CAD build for the part. Positions are in the model's coordinates, mm. A direction names the side the tool comes from. Give positions to 0.01 mm unless a question says otherwise; leave off trailing zeros. Write each loop counter-clockwise with the first axis right and the second up, starting at its lowest first coordinate (ties: lowest second). Pieces come first, ordered by that corner, then holes. Notation, with made-up numbers: (62, -9) - (75, -9) arc R26 cw to (75, 7) - close; hole circle Ø2 at (58, 22.25). An arc over 180 degrees is marked (long way). Put each result on its own line as item: value. Start each with the question number.
1. Cut at B-B on x = 16.25. List the corners of the cut face in (y, z).
2. Wall check: line 1 (Z direction, x = 14, y = 4); line 2 (Z direction, x = 14, y = 2); line 3 (X direction, y = 4, z = 29.25). Give the ranges that are in metal, low to high.
3. Cut at D-D on y = 4. List the corners of the cut face in (x, z), and give its area (4 significant figures).
4. Cut at A-A on y = 0.25. List the corners of the cut face in (x, z), and give its area (4 significant figures).
5. Mould opens along Y. For faces 5 (the flat face through (17.25, 4, 22)), 6 (the flat face through (15, 2, 28)), 7 (the flat face through (16, 4, 33)) say: +Y half, -Y half, draft (parallel to the pull), parting line (faces both ways), or undercut.
6. Cut at C-C on z = 23. List the corners of the cut face in (x, y), and give its area (4 significant figures).
7. Tool access for faces 1 (the flat face through (15, 0, 23)), 2 (the cylindrical face through (15.514, 6.285, 25.801)), 3 (the flat face through (13.75, 4, 22)), 4 (the flat face through (10, 4, 22)): list every direction of +Z, -Z, +X, -X, +Y, -Y with a clear straight run to the whole face (end or side of a thin tool).
8. Drop flat-ended pins along their axis: pin 1 (4.5 mm diameter, centred on x = 15, z = 23.5, fed in from -Y); pin 2 (1.8 mm diameter, centred on y = 2, z = 32, fed in from -X); pin 3 (1 mm diameter, centred on y = 4, z = 30.5, fed in from +X). Give the stop position or say it passes through.
Autodesk Fusion 360 part; units mm, degrees
sketch "Sketch1" plane through (0, 0, 0) normal (0, 1, 0) x (1, 0, 0)
  line L0 (10, -20) -> (21, -20)
  line L1 (21, -20) -> (21, -23.5)
  line L2 (21, -23.5) -> (24, -23.5)
  line L3 (24, -23.5) -> (24, -25.5)
  line L4 (24, -25.5) -> (7, -25.5)
  line L5 (7, -25.5) -> (7, -23.5)
  line L6 (7, -23.5) -> (10, -23.5)
  line L7 (10, -23.5) -> (10, -20)
extrude "Extrude1" add sketch "Sketch1" along normal blind 7.6
sketch "Sketch2" plane through (0, 0, 20) normal (0, 0, -1) x (1, 0, 0)
  line L0 (21, 0) -> (10, 0)
  line L1 (10, 0) -> (10, -7.6)
  line L2 (10, -7.6) -> (21, -7.6)
  line L3 (21, -7.6) -> (21, 0)
  line L4 (17.25, -2.05) -> (13.75, -2.05)
  line L5 (13.75, -2.05) -> (13.75, -5.55)
  line L6 (13.75, -5.55) -> (17.25, -5.55)
  line L7 (17.25, -5.55) -> (17.25, -2.05)
  line L8 (17.25, -2.05) -> (13.75, -5.55) construction
  line L9 (13.75, -2.05) -> (17.25, -5.55) construction
  point P0 (15.5, -3.8)
  dimension "d9" = 3.5
  dimension "d10" = 3.5
extrude "Extrude2" cut sketch "Sketch2" against normal blind 5 contours L4 L5 L6 L7
sketch "Sketch3" plane through (0, 0, 0) normal (0, 0, 1) x (1, 0, 0)
  line L0 (14, 0) -> (14.5, 0)
  line L1 (14.5, 0) -> (13.5, 0)
sketch "Sketch4" plane through (0, 0, 0) normal (0, -1, 0) x (1, 0, 0)
  line L0 (7, 23.5) -> (10, 23.5)
  line L1 (10, 23.5) -> (10, 20)
  line L2 (10, 20) -> (21, 20)
  line L3 (21, 20) -> (21, 23.5)
  line L4 (21, 23.5) -> (24, 23.5)
  line L5 (24, 23.5) -> (24, 25.5)
  line L6 (24, 25.5) -> (7, 25.5)
  line L7 (7, 25.5) -> (7, 23.5)
  line L8 (15.5, 25.5) -> (16.5, 25.5)
  line L9 (16.5, 25.5) -> (16.5, 29.5)
  line L10 (16.5, 29.5) -> (14.5, 29.5)
  line L11 (14.5, 29.5) -> (14.5, 25.5)
  line L12 (14.5, 25.5) -> (15.5, 25.5)
  line L13 (15.5, 29.5) -> (17.25, 29.5)
  line L14 (17.25, 29.5) -> (17.25, 33)
  line L15 (17.25, 33) -> (13.75, 33)
  line L16 (13.75, 33) -> (13.75, 29.5)
  line L17 (13.75, 29.5) -> (15.5, 29.5)
extrude "Extrude3" add sketch "Sketch4" against normal blind 4 from surface at -2 contours L6 L8 L9 L10 L11 L12 L13 L17
extrude "Extrude4" add sketch "Sketch4" against normal blind 10.5 from surface at 1.44 contours L10 L13 L14 L15 L16 L17
fillet "Fillet1" radius 1 8 edges at (15.5, -1.44, 29.5) (15.5, -1.44, 33) (15.5, 9.06, 33) (15.5, 9.06, 29.5) (15.5, 6, 29.5) (15.5, 2, 29.5) (15.5, 2, 25.5) (15.5, 6, 25.5)
Report:
1. outline: (-1.44, 30.5) arc R1 ccw to (-0.44, 29.5) - (1, 29.5) arc R1 cw to (2, 28.5) - (2, 26.5) arc R1 cw to (1, 25.5) - (0, 25.5) - (0, 20) - (2.05, 20) - (2.05, 25) - (5.55, 25) - (5.55, 20) - (7.6, 20) - (7.6, 25.5) - (7, 25.5) arc R1 cw to (6, 26.5) - (6, 28.5) arc R1 cw to (7, 29.5) - (8.06, 29.5) arc R1 ccw to (9.06, 30.5) - (9.06, 32) arc R1 ccw to (8.06, 33) - (-0.44, 33) arc R1 ccw to (-1.44, 32) - close
2. line 1: z = 25 to 25.5, 29.5 to 33
2. line 2: z = 20 to 25.5, 29.5 to 33
2. line 3: x = 14.5 to 16.5
3. outline: (7, 23.5) - (10, 23.5) - (10, 20) - (13.75, 20) - (13.75, 25) - (17.25, 25) - (17.25, 20) - (21, 20) - (21, 23.5) - (24, 23.5) - (24, 25.5) - (16.5, 25.5) - (16.5, 29.5) - (17.25, 29.5) - (17.25, 33) - (13.75, 33) - (13.75, 29.5) - (14.5, 29.5) - (14.5, 25.5) - (7, 25.5) - close
3. area: 75.25 mm²
4. outline: (7, 23.5) - (10, 23.5) - (10, 20) - (21, 20) - (21, 23.5) - (24, 23.5) - (24, 25.5) - (7, 25.5) - close; (13.75, 29.5) - (17.25, 29.5) - (17.25, 33) - (13.75, 33) - close
4. area: 84.75 mm²
5. face 5: undercut
5. face 6: -Y half
5. face 7: draft
6. outline: (10, 0) - (21, 0) - (21, 7.6) - (10, 7.6) - close; hole (13.75, 2.05) - (17.25, 2.05) - (17.25, 5.55) - (13.75, 5.55) - close
6. area: 71.35 mm²
7. face 1: -Z, +X, -X, -Y
7. face 2: +X, -X, +Y
7. face 3: -Z
7. face 4: -Z, -X, +Y, -Y
8. pin 1: stops at y = 0
8. pin 2: stops at x = 13.75
8. pin 3: stops at x = 17.25
